CAD build for the part. Positions are in the model's coordinates, mm. Face numbers are marked on the shaded views. A direction names the side the tool comes from. Give positions to 0.01 mm unless a question says otherwise; leave off trailing zeros. Loops run counter-clockwise (first coordinate to the right, second up) from the corner with the lowest first, then second, coordinate; pieces in that order, holes last.
```python
from build123d import *

# Parameters (mm, degrees)
SKETCH001_W     = 1.25
SKETCH001_H     = 6
PAD_DEPTH       = 20
PAD001_DEPTH    = 4
SKETCH003_W     = 7.25
SKETCH003_H     = 21
POCKET_DEPTH    = 5
SKETCH004_W     = 5
SKETCH004_H     = 8
PAD002_DEPTH    = 32.5
SKETCH005_R     = 1.75
SKETCH005_W     = 2.5
SKETCH005_H     = 8
POCKET001_DEPTH = 5
POCKET002_DEPTH = 30.055369


with BuildPart() as part:
    # Sketch → Revolution (revolve)
    with BuildSketch(Plane.XZ):
        Polygon((0, 0), (6.25, 0), (3.685308, 5.5), (3.685308, 14.5), (6.25, 20), (0, 20), align=None)
    revolve(axis=Axis((0, 0, 0), (0, 0, 1)))

    # Sketch001 → Pad (new body)
    with BuildSketch(Plane(origin=(0, 0, 20), x_dir=(-1, 0, 0), z_dir=(0, 0, 1))):
        with Locations((-1.625, 0)):
            Rectangle(SKETCH001_W, SKETCH001_H)
    extrude(amount=-PAD_DEPTH)

    # Sketch002 → Pad001 (new body)
    with BuildSketch(Plane.XZ.offset(3)):
        with BuildLine():
            Line((2.140443, 14.5), (10, 14.5))
            Line((10, 14.5), (10, 32.554369))
            Line((10, 32.554369), (21, 32.554369))
            Line((21, 32.554369), (45, 50))
            ThreePointArc((48.851141, 5.5), (53.111023, 28.285305), (45, 50))
            Line((45, 0), (48.851141, 5.5))
            Line((10, 0), (45, 0))
            Line((10, 5.5), (10, 0))
            Line((10, 5.5), (2.140443, 5.5))
            Line((2.140443, 5.5), (2.140443, 14.5))
        make_face()
    extrude(amount=-PAD001_DEPTH)

    # Sketch003 → Pocket (cut)
    with BuildSketch(Plane.XZ.offset(3)):
        with Locations((17.375, 19.554369)):
            Rectangle(SKETCH003_W, SKETCH003_H)
    extrude(amount=-POCKET_DEPTH, mode=Mode.SUBTRACT)

    # Sketch004 → Pad002 (new body)
    with BuildSketch(Plane(origin=(0, 0, 32.554369), x_dir=(-1, 0, 0), z_dir=(0, 0, 1))):
        with Locations((-11.25, 7)):
            Rectangle(SKETCH004_W, SKETCH004_H)
    extrude(amount=-PAD002_DEPTH)

    # Sketch005 → Pocket001 (cut)
    with BuildSketch(Plane(origin=(13.75, 0, 0), x_dir=(0, 0, 1), z_dir=(1, 0, 0))):
        with Locations((14.554369, 7)):
            Circle(SKETCH005_R)
        with Locations((24.554369, 7)):
            Circle(SKETCH005_R)
        Polygon((0.054369, 11), (13.910775, 11), (0.054369, 3), align=None)
        with Locations((31.304369, 7)):
            Rectangle(SKETCH005_W, SKETCH005_H)
    extrude(amount=-POCKET001_DEPTH, mode=Mode.SUBTRACT)

    # Sketch006 → Pocket002 (cut, through all)
    with BuildSketch(Plane(origin=(0, 0, 30.054369), x_dir=(-1, 0, 0), z_dir=(0, 0, 1))):
        Polygon((-10, 3), (-8.75, 3.721688), (-8.75, 3), align=None)
    extrude(amount=-POCKET002_DEPTH, mode=Mode.SUBTRACT)


solid = part.part
```
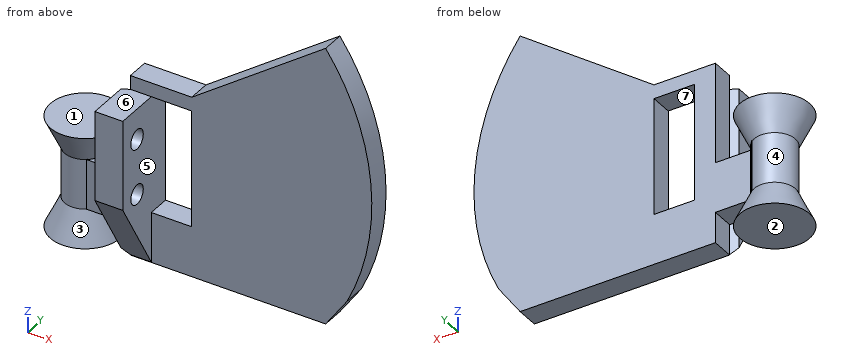
1. Drop flat-ended pins along their axis: pin 1 (13 mm diameter, centred on x = 33, z = 15, fed in from -Y); pin 2 (3 mm diameter, centred on x = 6.5, y = -1.5, fed in from +Z); pin 3 (8 mm diameter, centred on y = -5.5, z = 17.5, fed in from -X). Give the stop position or say it passes through.
Responses:
pin 1: stops at y = -3
pin 2: stops at z = 20
pin 3: stops at x = -5.78
2. Saw through at B-B, the plane y = 0. List the corners of the cut face in (x, z).
Responses:
outline: (-6.25, 0) - (6.25, 0) - (3.69, 5.5) - (10, 5.5) - (10, 0) - (45, 0) - (48.85, 5.5) arc R43.27 ccw to (45, 50) - (21, 32.55) - (10, 32.55) - (10, 14.5) - (3.69, 14.5) - (6.25, 20) - (-6.25, 20) - (-3.69, 14.5) - (-3.69, 5.5) - close; hole (13.75, 9.05) - (21, 9.05) - (21, 30.05) - (13.75, 30.05) - close
3. Tool access for the marked faces 4, 5, 6 and 7: list every direction of +Z, -Z, +X, -X, +Y, -Y with a clear straight run to the whole face (end or side of a thin tool).
Responses:
face 4: none
face 5: -Y
face 6: +Z, +X, -X, -Y
face 7: +Y, -Y
4. Pull direction Z, two halves, no side cores. Call the marked faces 1, 2 and 3: released by +Z, released by -Z, zero draft, split by the parting line, or undercut.
Responses:
face 1: released by +Z
face 2: released by -Z
face 3: undercut
5. Saw through at A-A, the plane x = 12.5. List the corners of the cut face in (y, z), and give its area (3 significant figures).
Responses:
outline: (-11, 13.91) - (-3, 0.05) - (-3, 0) - (1, 0) - (1, 32.55) - (-3, 32.55) - (-3, 30.05) - (-11, 30.05) - close; hole circle Ø3.5 at (-7, 14.55); hole circle Ø3.5 at (-7, 24.55)
area: 296 mm2
6. Saw through at C-C, the plane y = -7. List the corners of the cut face in (x, z).
Responses:
outline: (8.75, 6.98) - (13.75, 6.98) - (13.75, 12.8) - (8.75, 12.8) - close; (8.75, 16.3) - (13.75, 16.3) - (13.75, 22.8) - (8.75, 22.8) - close; (8.75, 26.3) - (13.75, 26.3) - (13.75, 30.05) - (8.75, 30.05) - close
7. Saw through at D-D, the plane x = 0. List the corners of the cut face in (y, z).
Responses:
outline: (-6.25, 0) - (6.25, 0) - (3.69, 5.5) - (3.69, 14.5) - (6.25, 20) - (-6.25, 20) - (-3.69, 14.5) - (-3.69, 5.5) - close
8. Probe line 1 along Z through (x, y) = (12.5, -7); line 2 along Y through (x, z) = (49, 11); line 3 along Z through (x, y) = (5.5, -0.75). List the from-to ranges inside material, lowest first.
Responses:
line 1: z = 6.98 to 12.8, 16.3 to 22.8, 26.3 to 30.05
line 2: y = -3 to 1
line 3: z = 0 to 1.5, 5.5 to 14.5, 18.5 to 20
